```python
from build123d import *

# Parameters (mm, degrees)
SKETCH1_R           = 4
SKETCH1_R_2         = 2.5
BOSS_EXTRUDE1_DEPTH = 9.6
CUT_EXTRUDE1_START  = -3.3
SKETCH2_R           = 2.5
CUT_EXTRUDE1_DEPTH  = 3.3
CUT_EXTRUDE2_DEPTH  = 228.086239125
SKETCH5_R           = 6
CUT_EXTRUDE3_DEPTH  = 5


with BuildPart() as part:
    # Sketch1 → Boss-Extrude1 (new body)
    with BuildSketch(Plane.XY):
        Polygon((221, 0), (5, 0), (0, -5), (0, -15), (5, -20), (221, -20), (226, -15), (226, -5), align=None)
        with Locations((38, -14)):
            Circle(SKETCH1_R, mode=Mode.SUBTRACT)
        with Locations((188, -14)):
            Circle(SKETCH1_R, mode=Mode.SUBTRACT)
        with Locations((16, -10)):
            Circle(SKETCH1_R_2, mode=Mode.SUBTRACT)
        with Locations((60, -10)):
            Circle(SKETCH1_R_2, mode=Mode.SUBTRACT)
        with BuildLine():
            ThreePointArc((98, -8.25), (100.5, -5.75), (103, -8.25))
            Line((103, -8.25), (103, -11.75))
            ThreePointArc((103, -11.75), (100.5, -14.25), (98, -11.75))
            Line((98, -11.75), (98, -8.25))
        make_face(mode=Mode.SUBTRACT)
        with BuildLine():
            Line((128, -8.25), (128, -11.75))
            ThreePointArc((128, -11.75), (125.5, -14.25), (123, -11.75))
            Line((123, -11.75), (123, -8.25))
            ThreePointArc((123, -8.25), (125.5, -5.75), (128, -8.25))
        make_face(mode=Mode.SUBTRACT)
        with Locations((166, -10)):
            Circle(SKETCH1_R_2, mode=Mode.SUBTRACT)
        with Locations((210, -10)):
            Circle(SKETCH1_R_2, mode=Mode.SUBTRACT)
    extrude(amount=BOSS_EXTRUDE1_DEPTH)

    # Sketch2 → Cut-Extrude1 (cut)
    # profile 1 of 2: a face of its own
    with BuildSketch(Plane.XY.offset(9.6).offset(CUT_EXTRUDE1_START)):
        with BuildLine():
            Line((48.392304845, -20), (113, -20))
            Line((113, -20), (113, 0))
            Line((113, 0), (5, 0))
            Line((5, 0), (0, -5))
            Line((0, -5), (0, -15))
            Line((0, -15), (5, -20))
            Line((5, -20), (27.607695155, -20))
            ThreePointArc((27.607695155, -20), (34.894171459, -2.408890085), (50, -14))
            ThreePointArc((50, -14), (49.591109915, -17.105828541), (48.392304845, -20))
        make_face()
        with Locations((16, -10)):
            Circle(SKETCH2_R, mode=Mode.SUBTRACT)
        with Locations((60, -10)):
            Circle(SKETCH2_R, mode=Mode.SUBTRACT)
        with BuildLine():
            Line((98, -11.75), (98, -8.25))
            ThreePointArc((98, -8.25), (100.5, -5.75), (103, -8.25))
            Line((103, -8.25), (103, -11.75))
            ThreePointArc((103, -11.75), (100.5, -14.25), (98, -11.75))
        make_face(mode=Mode.SUBTRACT)
    # profile 2 of 2: a face of its own
    with BuildSketch(Plane.XY.offset(9.6).offset(CUT_EXTRUDE1_START)):
        with BuildLine():
            Line((113, 0), (113, -20))
            Line((113, -20), (177.607695155, -20))
            ThreePointArc((177.607695155, -20), (184.894171459, -2.408890085), (200, -14))
            ThreePointArc((200, -14), (199.591109915, -17.105828541), (198.392304845, -20))
            Line((198.392304845, -20), (221, -20))
            Line((221, -20), (226, -15))
            Line((226, -15), (226, -5))
            Line((226, -5), (221, 0))
            Line((221, 0), (113, 0))
        make_face()
        with BuildLine():
            Line((123, -11.75), (123, -8.25))
            ThreePointArc((123, -8.25), (125.5, -5.75), (128, -8.25))
            Line((128, -8.25), (128, -11.75))
            ThreePointArc((128, -11.75), (125.5, -14.25), (123, -11.75))
        make_face(mode=Mode.SUBTRACT)
        with Locations((166, -10)):
            Circle(SKETCH2_R, mode=Mode.SUBTRACT)
        with Locations((210, -10)):
            Circle(SKETCH2_R, mode=Mode.SUBTRACT)
    extrude(amount=CUT_EXTRUDE1_DEPTH, mode=Mode.SUBTRACT)

    # Sketch4 → Cut-Extrude2 (cut, through all)
    with BuildSketch(Plane.XZ.offset(20)):
        Polygon((143, 1.8), (152, 6.3), (113, 6.3), (74, 6.3), (83, 1.8), align=None)
    extrude(amount=-CUT_EXTRUDE2_DEPTH, mode=Mode.SUBTRACT)

    # Sketch5 → Cut-Extrude3 (cut)
    with BuildSketch(Plane.XY.offset(6.3)):
        with Locations((16, -10)):
            Circle(SKETCH5_R)
        with Locations((60, -10)):
            Circle(SKETCH5_R)
        with Locations((166, -10)):
            Circle(SKETCH5_R)
        with Locations((210, -10)):
            Circle(SKETCH5_R)
    extrude(amount=-CUT_EXTRUDE3_DEPTH, mode=Mode.SUBTRACT)


solid = part.part
```
Model file for the job. Use its own axes, mm. A direction names the side the tool comes from. Coordinates: 2 decimals unless noted, no trailing zeros. Order: outer loops, then holes, each group sorted by start corner. A loop starts at its lowest first (then second) coordinate and runs counter-clockwise, first axis right, second up. Notation, with made-up numbers: (2, -27) - (45, -27) arc R15 ccw to (45, -21) - close; hole circle Ø1 at (69, 1). An arc over 180 degrees is marked (long way). Return JSON: item names as keys, results as strings. Group by question number.
1) Saw through at C-C, the plane x = 145. Write the cut outline in (y, z).
2) Tool access for faces 1 (the cylindrical face through (14, -11.5, 0.6)), 2 (the cylindrical face through (21.723, -8.198, 3.835)): list every direction of +Z, -Z, +X, -X, +Y, -Y with a clear straight run to the whole face (end or side of a thin tool).
3) Saw through at D-D, the plane x = 92. Write the cut outline in (y, z), plus the area to 3 significant figures.
4) Saw through at B-B, the plane x = 38. Write the cut outline in (y, z), plus the area to 3 significant figures.
5) Mould opens along Y. For faces 3 (the flat face through (19, -10, 1.3)), 4 (the flat face through (147.4, -10.1, 4)), 5 (the flat face through (111.5, -20, 1.5)) say: released by +Y, released by -Y, zero draft, split by the parting line, or undercut.
6) Flat gauge pins, fed straight in: P1, Ø4.5, axis at x = 16, y = -10, coming from the +Z side; P2, Ø1.5, axis at x = 168, y = -17, coming from the +Z side; P3, Ø3, axis at x = 91, y = -17.5, coming from the +Z side; P4, Ø3.5, axis at x = 62.5, y = -10, coming from the +Z side. Where does each tip first touch, or does it go through?
7) Probe line 1 (X direction, y = -14.5, z = 7.5); line 2 (Y direction, x = 210, z = 0.35); line 3 (X direction, y = -8.5, z = 5.5). List the from-to ranges inside material, lowest first. Write a range as from..to.
8) Saw through at A-A, the plane x = 210. Write the cut outline in (y, z).
Values found:
{
 "1": {"outline": "(-20, 0) - (0, 0) - (0, 2.8) - (-20, 2.8) - close"},
 "2": {"face 1": "+Z, -Z", "face 2": "+Z"},
 "3": {"outline": "(-20, 0) - (0, 0) - (0, 1.8) - (-20, 1.8) - close", "area": "36.0 mm²"},
 "4": {"outline": "(-20, 0) - (-18, 0) - (-18, 9.6) - (-20, 9.6) - close; (-10, 0) - (0, 0) - (0, 6.3) - (-2, 6.3) - (-2, 9.6) - (-10, 9.6) - close", "area": "109 mm²"},
 "5": {"face 3": "undercut", "face 4": "zero draft", "face 5": "released by -Y"},
 "6": {"P1": "passes through", "P2": "stops at z = 6.3", "P3": "stops at z = 1.8", "P4": "stops at z = 1.3"},
 "7": {"line 1": "x = 26.01..34.03, 41.97..49.99, 176.01..184.03, 191.97..199.99", "line 2": "y = -20..-12.5, -7.5..0", "line 3": "x = 0..10.19, 21.81..54.19, 65.81..75.6, 150.4..160.19, 171.81..204.19, 215.81..226"},
 "8": {"outline": "(-20, 0) - (-12.5, 0) - (-12.5, 1.3) - (-16, 1.3) - (-16, 6.3) - (-20, 6.3) - close; (-7.5, 0) - (0, 0) - (0, 6.3) - (-4, 6.3) - (-4, 1.3) - (-7.5, 1.3) - close"}
}
